Print and shaded views of the part. All mm, measured from the part's lowest x, y and z. Coordinates: 2 decimals unless noted, no trailing zeros. Order: outer loops, then holes, each group sorted by start corner. A loop starts at its lowest first (then second) coordinate and runs counter-clockwise, first axis right, second up. Notation, with made-up numbers: M 83,60.25 L 120,60.25 A24 ccw 120,86.25 Z; hole C 19,-28 d4. An arc over 180 degrees is marked long. One line per item, written item: value.
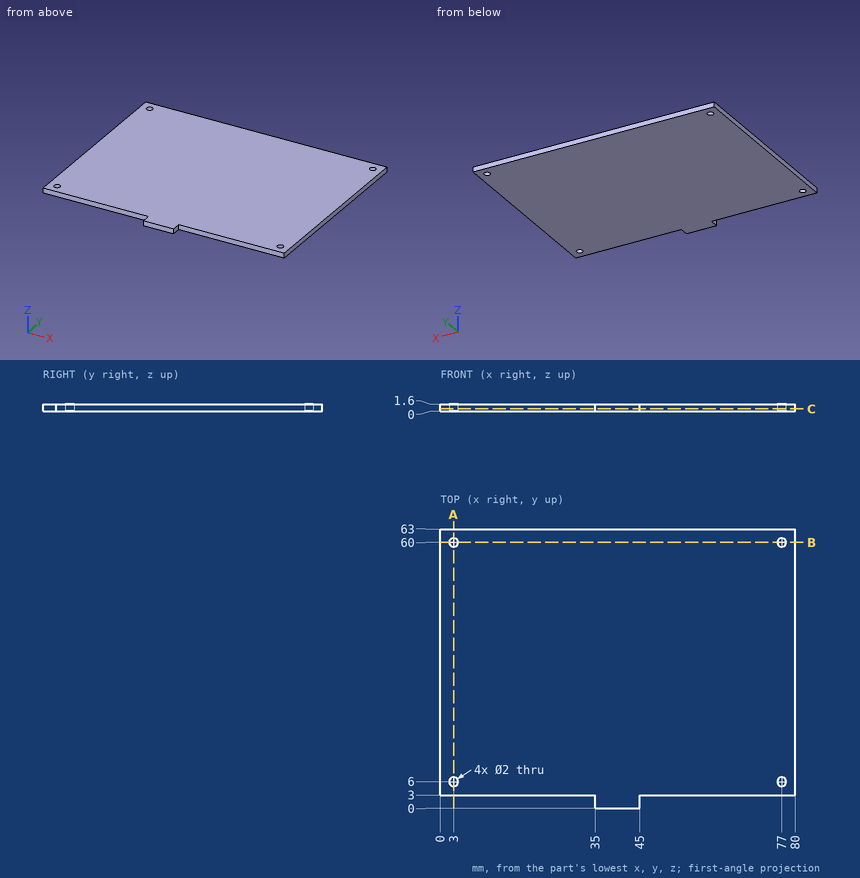
Q1. Slice it at B-B (y = 60). List the corners of the cut face in (x, z).
Recorded:
outline: M 0,0 L 2,0 L 2,1.6 L 0,1.6 Z; M 4,0 L 76,0 L 76,1.6 L 4,1.6 Z; M 78,0 L 80,0 L 80,1.6 L 78,1.6 Z
Q2. Drill centre lines: line 1 along Y through (x, z) = (3, 1.2); line 2 along Y through (x, z) = (57, 1.3). Where is each one in solid material? Low to high.
Recorded:
line 1: y = 3 to 5, 7 to 59, 61 to 63
line 2: y = 3 to 63
Q3. Slice it at A-A (x = 3). List the corners of the cut face in (y, z), plus the area to 3 significant figures.
Recorded:
outline: M 3,0 L 5,0 L 5,1.6 L 3,1.6 Z; M 7,0 L 59,0 L 59,1.6 L 7,1.6 Z; M 61,0 L 63,0 L 63,1.6 L 61,1.6 Z
area: 89.6 mm^2
Q4. Slice it at C-C (z = 0.5). List the corners of the cut face in (x, y), plus the area to 3 significant figures.
Recorded:
outline: M 0,3 L 35,3 L 35,0 L 45,0 L 45,3 L 80,3 L 80,63 L 0,63 Z; hole C 3,6 d2; hole C 3,60 d2; hole C 77,6 d2; hole C 77,60 d2
area: 4,820 mm^2
Q5. Pin check, flat tips, straight feed: pin 1 Ø1 at (x, y) = (12, 31.5) entering from -Z; pin 2 Ø0.5 at (x, z) = (67.5, 0.5) entering from -Y. Stop position of each tip, or through.
Recorded:
pin 1: stops at z = 0
pin 2: stops at y = 3
